Autodesk Fusion 360 part; units mm, degrees
sketch "Sketch1" plane through (0, 0, 0) normal (0, 0, 1) x (1, 0, 0)
  line L0 (0, 0) -> (84, 0)
  line L1 (84, 0) -> (84, 60)
  line L2 (84, 60) -> (0, 60)
  line L3 (0, 60) -> (0, 0)
  line L4 (5, 60) -> (5, 0) construction
  line L5 (79, 60) -> (79, 0) construction
  line L6 (5, 50) -> (79, 50) construction
  line L7 (5, 10) -> (79, 10) construction
  line L8 (7.75, 50) -> (7.75, 10) construction
  line L9 (76.25, 50) -> (76.25, 10) construction
  line L10 (5, 55) -> (79, 55) construction
  line L11 (5, 5) -> (79, 5) construction
  line L12 (7.75, 10) -> (7.75, 5) construction
  line L13 (7.75, 50) -> (7.75, 55) construction
  line L14 (76.25, 50) -> (76.25, 55) construction
  line L15 (76.25, 10) -> (76.25, 5) construction
  line L16 (7.75, 15) -> (76.25, 15) construction
  line L17 (7.75, 45) -> (76.25, 45) construction
  line L18 (5, 55) -> (5, 45)
  arc A0 (5, 45) -> (10.5, 45) centre (7.75, 45) ccw
  line L19 (10.5, 45) -> (10.5, 55)
  arc A1 (10.5, 55) -> (5, 55) centre (7.75, 55) ccw
  line L20 (7.75, 55) -> (7.75, 45) construction
  line L21 (10.5, 5) -> (10.5, 15)
  arc A2 (10.5, 15) -> (5, 15) centre (7.75, 15) ccw
  line L22 (5, 15) -> (5, 5)
  arc A3 (5, 5) -> (10.5, 5) centre (7.75, 5) ccw
  line L23 (7.75, 5) -> (7.75, 15) construction
  line L24 (73.5, 55) -> (73.5, 45)
  arc A4 (73.5, 45) -> (79, 45) centre (76.25, 45) ccw
  line L25 (79, 45) -> (79, 55)
  arc A5 (79, 55) -> (73.5, 55) centre (76.25, 55) ccw
  line L26 (76.25, 55) -> (76.25, 45) construction
  line L27 (73.5, 15) -> (73.5, 5)
  arc A6 (73.5, 5) -> (79, 5) centre (76.25, 5) ccw
  line L28 (79, 5) -> (79, 15)
  arc A7 (79, 15) -> (73.5, 15) centre (76.25, 15) ccw
  line L29 (76.25, 15) -> (76.25, 5) construction
  line L30 (15.5, 55) -> (68.5, 55)
  line L31 (68.5, 55) -> (68.5, 5)
  line L32 (68.5, 5) -> (15.5, 5)
  line L33 (15.5, 5) -> (15.5, 55)
  line L34 (15.5, 55) -> (68.5, 5) construction
  line L35 (68.5, 55) -> (15.5, 5) construction
  line L36 (68.5, 55) -> (68.5, 5) construction
  line L37 (15.5, 55) -> (15.5, 5) construction
  line L38 (50, 15) -> (50, 45) construction
  line L39 (34, 15) -> (34, 45) construction
  line L40 (31.9215, 18.6) -> (29.8431, 15)
  line L41 (29.8431, 15) -> (31.9215, 11.4)
  line L42 (31.9215, 11.4) -> (36.0785, 11.4)
  line L43 (36.0785, 11.4) -> (38.1569, 15)
  line L44 (38.1569, 15) -> (36.0785, 18.6)
  line L45 (36.0785, 18.6) -> (31.9215, 18.6)
  line L46 (36.0785, 41.4) -> (38.1569, 45)
  line L47 (38.1569, 45) -> (36.0785, 48.6)
  line L48 (36.0785, 48.6) -> (31.9215, 48.6)
  line L49 (31.9215, 48.6) -> (29.8431, 45)
  line L50 (29.8431, 45) -> (31.9215, 41.4)
  line L51 (31.9215, 41.4) -> (36.0785, 41.4)
  line L52 (52.0785, 41.4) -> (54.1569, 45)
  line L53 (54.1569, 45) -> (52.0785, 48.6)
  line L54 (52.0785, 48.6) -> (47.9215, 48.6)
  line L55 (47.9215, 48.6) -> (45.8431, 45)
  line L56 (45.8431, 45) -> (47.9215, 41.4)
  line L57 (47.9215, 41.4) -> (52.0785, 41.4)
  line L58 (47.9215, 18.6) -> (45.8431, 15)
  line L59 (45.8431, 15) -> (47.9215, 11.4)
  line L60 (47.9215, 11.4) -> (52.0785, 11.4)
  line L61 (52.0785, 11.4) -> (54.1569, 15)
  line L62 (54.1569, 15) -> (52.0785, 18.6)
  line L63 (52.0785, 18.6) -> (47.9215, 18.6)
  point P0 (42, 30)
  point P1 (34, 15)
  point P2 (34, 45)
  point P3 (50, 45)
  point P4 (50, 15)
  dimension "d1" = 84
  dimension "d2" = 60
  dimension "d3" = 5
  dimension "d4" = 5
  dimension "d5" = 2.75
  dimension "d6" = 2.75
  dimension "d7" = 40
  dimension "d8" = 5
  dimension "d9" = 5
  dimension "d10" = 5
  dimension "d11" = 5
  dimension "d12" = 5.5
  dimension "d13" = 5.5
  dimension "d16" = 53
  dimension "d17" = 50
  dimension "d18" = 18.5
  dimension "d19" = 18.5
  dimension "d20" = 3.6
  dimension "d21" = 3.6
  dimension "d22" = 3.6
  dimension "d23" = 3.6
extrude "Extrude1" add sketch "Sketch1" against normal blind 5.3 contours L0 L1 L2 L3 | L30 L31 L32 L33
extrude "Extrude2" add sketch "Sketch1" along normal blind 0.2 contours L30 L31 L32 L33 | L40 L41 L42 L43 L44 L45 | L46 L47 L48 L49 L50 L51 | L52 L53 L54 L55 L56 L57 | L58 L59 L60 L61 L62 L63
sketch "Sketch2" plane through (0, 0, 0.2) normal (0, 0, 1) x (-1, 0, 0)
  line L0 (-15.5, -5) -> (-68.5, -5)
  line L1 (-68.5, -5) -> (-68.5, -55)
  line L2 (-68.5, -55) -> (-15.5, -55)
  line L3 (-15.5, -55) -> (-15.5, -5)
  circle A0 centre (-34, -45) radius 2.1
  circle A1 centre (-50, -45) radius 2.1
  circle A2 centre (-34, -15) radius 2.1
  circle A3 centre (-50, -15) radius 2.1
  point P0 (-50, -45)
  point P1 (-34, -45)
  point P2 (-34, -15)
  point P3 (-50, -15)
  dimension "d26" = 4.2
  dimension "d27" = 4.2
  dimension "d28" = 4.2
  dimension "d29" = 4.2
extrude "Extrude3" add sketch "Sketch2" along normal blind 3.5
Check sheet for the modelled part. Datum: model origin and axes. Units: mm. A direction names the side the tool comes from. Round coordinates to 2 decimals unless told otherwise and drop trailing zeros. Order: outer loops, then holes, each group sorted by start corner. A loop starts at its lowest first (then second) coordinate and runs counter-clockwise, first axis right, second up.
Q1. Set-up check for faces 4 (the face through (42, 5, 2)), 5 (the face through (34, 45, 0.2)), 6 (the face through (42, 55, 2)), 7 (the face through (34, 18.6, -3)): record each of +Z, -Z, +X, -X, +Y, -Y from which the full face is reachable in a straight line by a thin tool's end or side.
Filled sheet:
face 4: +Z, +X, -X, -Y
face 5: +Z
face 6: +Z, +X, -X, +Y
face 7: -Z
Q2. Depth check by flat-ended pin: P1, Ø4, axis at x = 10.5, y = 52.5, coming from the +Z side; P2, Ø2, axis at x = 50, y = 46, coming from the -Z side; P3, Ø1.3, axis at x = 34.5, y = 45, coming from the +Z side. Enter the tip coordinate at first touch or a pass-through.
Filled sheet:
P1: stops at z = 0
P2: stops at z = 0
P3: stops at z = 0.2
Q3. Scan lines: L1, parallel to X at y = 45, z = 1.9; L2, parallel to Y at x = 50, z = 2.7; L3, parallel to X at y = 55, z = -2.75. Record each from-to range of solid material in increasing order.
Filled sheet:
L1: x = 15.5 to 31.9, 36.1 to 47.9, 52.1 to 68.5
L2: y = 5 to 12.9, 17.1 to 42.9, 47.1 to 55
L3: x = 0 to 5, 10.5 to 73.5, 79 to 84
Q4. Cross-section at C-C, the plane x = 76.25. Enter the section's corners in (y, z), plus the area to 3 significant figures.
Filled sheet:
outline: (0, -5.3) - (2.25, -5.3) - (2.25, 0) - (0, 0) - close; (17.75, -5.3) - (42.25, -5.3) - (42.25, 0) - (17.75, 0) - close; (57.75, -5.3) - (60, -5.3) - (60, 0) - (57.75, 0) - close
area: 154 mm2
Q5. Cross-section at A-A, the plane y = 9. Enter the section's corners in (x, z), plus the area to 3 significant figures.
Filled sheet:
outline: (0, -5.3) - (5, -5.3) - (5, 0) - (0, 0) - close; (10.5, -5.3) - (73.5, -5.3) - (73.5, 0) - (68.5, 0) - (68.5, 3.7) - (15.5, 3.7) - (15.5, 0) - (10.5, 0) - close; (79, -5.3) - (84, -5.3) - (84, 0) - (79, 0) - close
area: 583 mm2
Q6. Draft check along Y on faces 1 (the face through (43, 60, -3)), 2 (the face through (34, 45, 0)), 3 (the face through (41, 30, -5.3)). Enter one of: pulls with the +Y half, pulls with the -Y half, needs draft (parallel to the pull), parting line crosses it, or undercut.
Filled sheet:
face 1: pulls with the +Y half
face 2: undercut
face 3: needs draft
Q7. Cross-section at B-B, the plane z = 2.5. Enter the section's corners in (x, y), plus the area to 3 significant figures.
Filled sheet:
outline: (15.5, 5) - (68.5, 5) - (68.5, 55) - (15.5, 55) - close; hole circle Ø4.2 at (34, 15); hole circle Ø4.2 at (34, 45); hole circle Ø4.2 at (50, 15); hole circle Ø4.2 at (50, 45)
area: 2,590 mm2
Q8. Cross-section at D-D, the plane x = 34. Enter the section's corners in (y, z), plus the area to 3 significant figures.
Filled sheet:
outline: (0, -5.3) - (11.4, -5.3) - (11.4, 0) - (18.6, 0) - (18.6, -5.3) - (41.4, -5.3) - (41.4, 0) - (48.6, 0) - (48.6, -5.3) - (60, -5.3) - (60, 0) - (55, 0) - (55, 3.7) - (47.1, 3.7) - (47.1, 0.2) - (42.9, 0.2) - (42.9, 3.7) - (17.1, 3.7) - (17.1, 0.2) - (12.9, 0.2) - (12.9, 3.7) - (5, 3.7) - (5, 0) - (0, 0) - close
area: 397 mm2
